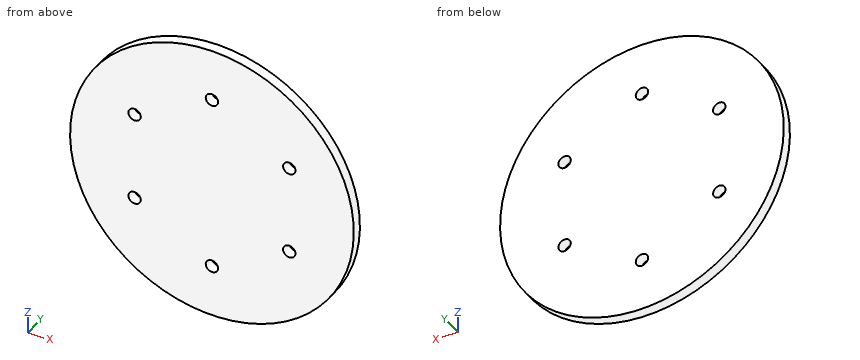
```python
from build123d import *

# Parameters (mm, degrees)
SKETCH1_R           = 67.5
BOSS_EXTRUDE1_DEPTH = 2.5
SKETCH2_R           = 2.95
CUT_EXTRUDE1_DEPTH  = 5


with BuildPart() as part:
    # Sketch1 → Boss-Extrude1 (new, symmetric)
    with BuildSketch(Plane(origin=(0, 0, 0), x_dir=(1, 0, 0), z_dir=(0, 1, 0))):
        with Locations(Location((0, 0, 0), (0, 0, 270))):
            Circle(SKETCH1_R)
    extrude(amount=BOSS_EXTRUDE1_DEPTH, both=True)

    # Sketch2 → Cut-Extrude1 (cut)
    with BuildSketch(Plane(origin=(0, 2.5, 0), x_dir=(1, 0, 0), z_dir=(0, 1, 0))):
        with Locations(Location((0, 42.5, 0), (0, 0, 270))):
            Circle(SKETCH2_R)
        with Locations(Location((36.806079661, 21.25, 0), (0, 0, 270))):
            Circle(SKETCH2_R)
        with Locations(Location((36.806079661, -21.25, 0), (0, 0, 270))):
            Circle(SKETCH2_R)
        with Locations(Location((0, -42.5, 0), (0, 0, 270))):
            Circle(SKETCH2_R)
        with Locations(Location((-36.806079661, -21.25, 0), (0, 0, 270))):
            Circle(SKETCH2_R)
        with Locations(Location((-36.806079661, 21.25, 0), (0, 0, 270))):
            Circle(SKETCH2_R)
    extrude(amount=-CUT_EXTRUDE1_DEPTH, mode=Mode.SUBTRACT)


solid = part.part
```
Source: CAD feature listing. Evaluate the final solid. Frame: model axes, mm. Coordinates: 2 decimals unless noted, no trailing zeros. Write each loop counter-clockwise with the first axis right and the second up, starting at its lowest first coordinate (ties: lowest second). Pieces come first, ordered by that corner, then holes. Notation, with made-up numbers: (-6, 52) -> (9, 52) arc R16 ccw to (9, 72) -> close; hole circle Ø11 at (72, -28). An arc over 180 degrees is marked (long way). Return JSON: item names as keys, results as strings. Group by question number.
1) Section query A-A, the plane x = 0. Return loops of the section in (y, z).
2) Contact query for flat-ended pins moving along their axis: P1, Ø7, axis at x = 36.81, z = 21.25, coming from the +Y side; P2, Ø1, axis at x = -35.5, y = 1.5, coming from the -Z side; P3, Ø2, axis at x = 4.5, y = 1, coming from the -Z side; P4, Ø5.5, axis at x = -36.81, z = 21.25, coming from the +Y side. Output: stop coordinate, or through.
3) Section query B-B, the plane z = -21.25. Return loops of the section in (x, y), plus the area to 3 significant figures.
4) Ray query, line 1 along X through (y, z) = (1, -21.25); line 2 along Z through (x, y) = (-2, 1.65); line 3 along Z through (x, y) = (-2.5, -1.1). Return the intervals inside material, ascending.
5) Section query C-C, the plane y = -1.05. Return loops of the section in (x, z).
6) Section query D-D, the plane z = -42.5. Return loops of the section in (x, y), plus the area to 3 significant figures.
From the geometry:
{
 "1": {"outline": "(-2.5, -67.5) -> (2.5, -67.5) -> (2.5, -45.45) -> (-2.5, -45.45) -> close; (-2.5, -39.55) -> (2.5, -39.55) -> (2.5, 39.55) -> (-2.5, 39.55) -> close; (-2.5, 45.45) -> (2.5, 45.45) -> (2.5, 67.5) -> (-2.5, 67.5) -> close"},
 "2": {"P1": "y = 2.5", "P2": "z = -57.72", "P3": "z = -67.41", "P4": "through"},
 "3": {"outline": "(-64.07, -2.5) -> (-39.76, -2.5) -> (-39.76, 2.5) -> (-64.07, 2.5) -> close; (-33.86, -2.5) -> (33.86, -2.5) -> (33.86, 2.5) -> (-33.86, 2.5) -> close; (39.76, -2.5) -> (64.07, -2.5) -> (64.07, 2.5) -> (39.76, 2.5) -> close", "area": "582 mm²"},
 "4": {"line 1": "-64.07 to -39.76, -33.86 to 33.86, 39.76 to 64.07", "line 2": "-67.47 to -44.67, -40.33 to 40.33, 44.67 to 67.47", "line 3": "-67.45 to -44.07, -40.93 to 40.93, 44.07 to 67.45"},
 "5": {"outline": "circle Ø135 at (0, 0); hole circle Ø5.9 at (-36.81, -21.25); hole circle Ø5.9 at (-36.81, 21.25); hole circle Ø5.9 at (0, -42.5); hole circle Ø5.9 at (0, 42.5); hole circle Ø5.9 at (36.81, -21.25); hole circle Ø5.9 at (36.81, 21.25)"},
 "6": {"outline": "(-52.44, -2.5) -> (-2.95, -2.5) -> (-2.95, 2.5) -> (-52.44, 2.5) -> close; (2.95, -2.5) -> (52.44, -2.5) -> (52.44, 2.5) -> (2.95, 2.5) -> close", "area": "495 mm²"}
}
